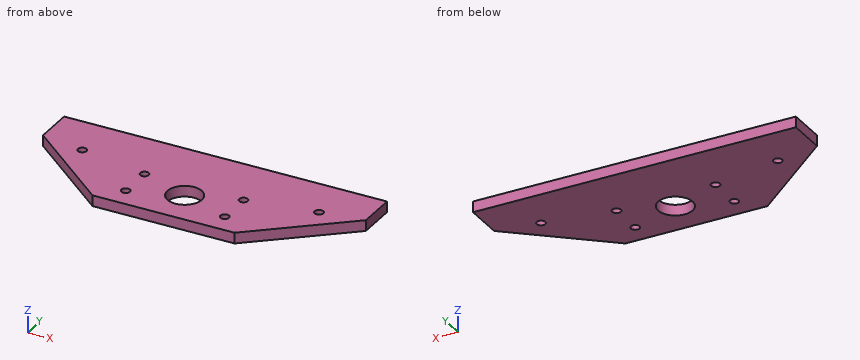
from build123d import *

# Parameters (mm, degrees)
SKETCH_1_W          = 150
SKETCH_1_H          = 70
EXTRUDE_1_DEPTH     = 5
SKETCH_2_R          = 8
CUT_EXTRUDE_1_DEPTH = 83.949769328
SKETCH_3_R          = 2
CUT_EXTRUDE_2_DEPTH = 83.949769328
SKETCH_4_R          = 2
CUT_EXTRUDE_3_DEPTH = 83.949769328
CUT_EXTRUDE_4_DEPTH = 83.949769328


with BuildPart() as part:
    # 스케치1 → 보스-돌출1 (new body)
    with BuildSketch(Plane.XY):
        with Locations((0, -0.080824272)):
            Rectangle(SKETCH_1_W, SKETCH_1_H)
    extrude(amount=EXTRUDE_1_DEPTH)

    # 스케치2 → 컷-돌출1 (cut, through all)
    with BuildSketch(Plane.XY.offset(5)):
        Circle(SKETCH_2_R)
    extrude(amount=-CUT_EXTRUDE_1_DEPTH, mode=Mode.SUBTRACT)

    # 스케치3 → 컷-돌출2 (cut, through all)
    with BuildSketch(Plane.XY.offset(5)):
        with Locations((-23, 8)):
            Circle(SKETCH_3_R)
        with Locations(Location((-23, -8, 0), (0, 0, 180))):
            Circle(SKETCH_3_R)
        with Locations((23, -8)):
            Circle(SKETCH_3_R)
        with Locations(Location((23, 8, 0), (0, 0, 180))):
            Circle(SKETCH_3_R)
    extrude(amount=-CUT_EXTRUDE_2_DEPTH, mode=Mode.SUBTRACT)

    # 스케치4 → 컷-돌출3 (cut, through all)
    with BuildSketch(Plane.XY.offset(5)):
        with Locations((-55, 13.64900919)):
            Circle(SKETCH_4_R)
        with Locations((-65, -25.080824272)):
            Circle(SKETCH_4_R)
        with Locations(Location((65, -25.080824272, 0), (0, 0, 180))):
            Circle(SKETCH_4_R)
        with Locations(Location((55, 13.64900919, 0), (0, 0, 180))):
            Circle(SKETCH_4_R)
    extrude(amount=-CUT_EXTRUDE_3_DEPTH, mode=Mode.SUBTRACT)

    # 스케치5 → 컷-돌출4 (cut, through all)
    with BuildSketch(Plane.XY.offset(5)):
        Polygon((-75, 16.919175728), (-33, -18), (33, -18), (75, 16.919175728), (75, -35.080824272), (-75, -35.080824272), (-75, -27.080824272), align=None)
    extrude(amount=-CUT_EXTRUDE_4_DEPTH, mode=Mode.SUBTRACT)


solid = part.part
Can you work these out from the model? Positions are in its coordinate system, mm. Give positions to 0.01 mm unless a question says otherwise; leave off trailing zeros. Loops run counter-clockwise (first coordinate to the right, second up) from the corner with the lowest first, then second, coordinate; pieces in that order, holes last. Notation, with made-up numbers: (65, 47) - (96, 47) arc R16 cw to (96, 60) - close; hole circle Ø10 at (-33, 38). An arc over 180 degrees is marked (long way). Answer as a JSON object with one key per item and string values.
Q1. Imagine slicing it at A-A on x = -23. Write out the boundary of the cut face in (y, z).
Geometry says:
{"outline": "(-18, 0) - (-10, 0) - (-10, 5) - (-18, 5) - close; (-6, 0) - (6, 0) - (6, 5) - (-6, 5) - close; (10, 0) - (34.92, 0) - (34.92, 5) - (10, 5) - close"}
Q2. Imagine slicing it at B-B on x = 0. Write out the boundary of the cut face in (y, z).
Geometry says:
{"outline": "(-18, 0) - (-8, 0) - (-8, 5) - (-18, 5) - close; (8, 0) - (34.92, 0) - (34.92, 5) - (8, 5) - close"}
Q3. Will these pins go through, and if not, where does the flat tip stop? P1, Ø2.5, axis at x = 55, y = 13.65, coming from the -Z side; P2, Ø2, axis at y = -11, z = 4, coming from the -X side.
Geometry says:
{"P1": "through", "P2": "x = -42.62"}
Q4. Imagine slicing it at D-D on z = 1.55. Write out the boundary of the cut face in (x, y).
Geometry says:
{"outline": "(-75, 16.92) - (-33, -18) - (33, -18) - (75, 16.92) - (75, 34.92) - (-75, 34.92) - close; hole circle Ø4 at (-55, 13.65); hole circle Ø4 at (-23, -8); hole circle Ø4 at (-23, 8); hole circle Ø16 at (0, 0); hole circle Ø4 at (23, -8); hole circle Ø4 at (23, 8); hole circle Ø4 at (55, 13.65)"}
Q5. Imagine slicing it at C-C on y = 3. Write out the boundary of the cut face in (x, z).
Geometry says:
{"outline": "(-58.26, 0) - (-7.42, 0) - (-7.42, 5) - (-58.26, 5) - close; (7.42, 0) - (58.26, 0) - (58.26, 5) - (7.42, 5) - close"}
Q6. If I drill on L1, parallel to Y at x = -23, z = 1.1; L2, parallel to Y at x = 0, z = 3.9; L3, parallel to X at y = 14, z = 4.75, over which ranges is the centre line in solid material (lowest first)?
Geometry says:
{"L1": "-18 to -10, -6 to 6, 10 to 34.92", "L2": "-18 to -8, 8 to 34.92", "L3": "-71.49 to -56.97, -53.03 to 53.03, 56.97 to 71.49"}
